Check sheet for the modelled part. Datum: model origin and axes. Units: mm. Face numbers are marked on the shaded views. Give positions to 0.01 mm unless a question says otherwise; leave off trailing zeros. Write each loop counter-clockwise with the first axis right and the second up, starting at its lowest first coordinate (ties: lowest second). Pieces come first, ordered by that corner, then holes. Notation, with made-up numbers: (32.5, 75) -> (59.5, 75) arc R28 ccw to (59.5, 110) -> close; hole circle Ø1 at (87, -1.75). An arc over 180 degrees is marked (long way). Return JSON: item names as keys, results as strings.
from build123d import *

# Parameters (mm, degrees)
F0_W     = 4
F0_H     = 6
F1_DEPTH = 28
F2_R     = 2
F3_DEPTH = 6
F4_R     = 1
F5_DEPTH = 1.1


# Not quite as in the source:
# - a feature names something its author has since deleted; it is built from what else it names


with BuildPart() as f1:
    # F0 (on Front) → F1 (new body)
    with BuildSketch(Plane.XZ):
        Rectangle(F0_W, F0_H)
    extrude(amount=F1_DEPTH)

    # F2 (on face) → F3 (join)
    with BuildSketch(Plane.YZ.offset(2)):
        with Locations((-4, 0)):
            Circle(F2_R)
    extrude(amount=F3_DEPTH)

    # F4 (on face) → F5 (join)
    with BuildSketch(Plane.XZ.offset(28)):
        Circle(F4_R)
    extrude(amount=F5_DEPTH)


solid = f1.part
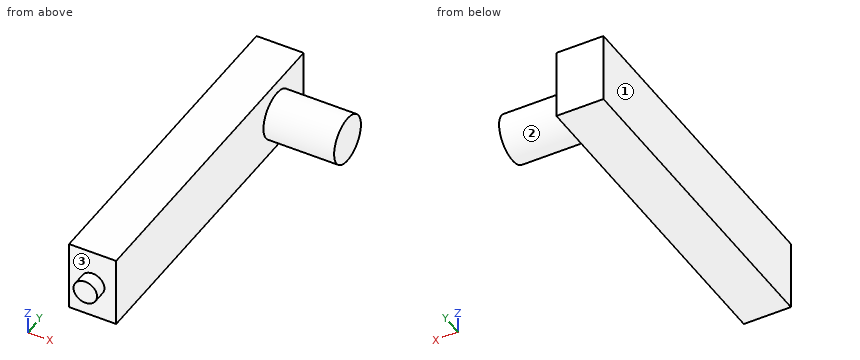
(1) Cross-section at C-C on x = 0. Enter the section's corners in (y, z).
Reply:
{"outline": "(-29.1, -1) -> (-28, -1) -> (-28, -3) -> (0, -3) -> (0, 3) -> (-28, 3) -> (-28, 1) -> (-29.1, 1) -> close"}
(2) Cross-section at A-A on y = -4. Enter the section's corners in (x, z).
Reply:
{"outline": "(-2, -3) -> (2, -3) -> (2, -2) -> (8, -2) -> (8, 2) -> (2, 2) -> (2, 3) -> (-2, 3) -> close"}
(3) Cross-section at D-D on x = 1.5. Enter the section's corners in (y, z).
Reply:
{"outline": "(-28, -3) -> (0, -3) -> (0, 3) -> (-28, 3) -> close"}
(4) Depth check by flat-ended pin: pin 1 Ø3 at (y, z) = (-11.5, -0.5) entering from +X; pin 2 Ø3 at (x, z) = (4, 0) entering from -Y; pin 3 Ø1 at (x, z) = (4.5, 1) entering from +Y; pin 4 Ø6 at (x, y) = (5.5, -13) entering from -Z. Enter the tip coordinate at first touch or a pass-through.
Reply:
{"pin 1": "x = 2", "pin 2": "y = -6", "pin 3": "y = -2.06", "pin 4": "through"}
(5) Cross-section at B-B on z = 0. Enter the section's corners in (x, y).
Reply:
{"outline": "(-2, -28) -> (-1, -28) -> (-1, -29.1) -> (1, -29.1) -> (1, -28) -> (2, -28) -> (2, -6) -> (8, -6) -> (8, -2) -> (2, -2) -> (2, 0) -> (-2, 0) -> close"}
(6) Thickness scan on L1, parallel to X at y = -20.5, z = 0.5; L2, parallel to Y at x = -1, z = -1.7; L3, parallel to Y at x = 3, z = -1.45. Record the ranges inside material, lowest first.
Reply:
{"L1": "-2 to 2", "L2": "-28 to 0", "L3": "-5.38 to -2.62"}
(7) Release check for a two-part mould opening along Y. For the marked faces 1, 2 and 3 record: pulls with the +Y half, pulls with the -Y half, needs draft (parallel to the pull), parting line crosses it, or undercut.
Reply:
{"face 1": "needs draft", "face 2": "parting line crosses it", "face 3": "pulls with the -Y half"}
